from build123d import *

# Parameters (mm, degrees)
F0_R     = 65
F1_DEPTH = 174
F2_SIZE2 = 60
F2_SIZE  = 7
F3_R     = 1
F4_R     = 10
F5_R     = 66.5
F5_R_2   = 65
F6_DEPTH = 6
F7_R     = 1


with BuildPart() as f1:
    # F0 (on Top) → F1 (new body)
    with BuildSketch(Plane.XY):
        Circle(F0_R)
    extrude(amount=-F1_DEPTH)

    # F2
    f2_edges = [f1.edges().sort_by_distance(p)[0] for p in [
        (-65, 0, -174),
    ]]
    f2_side = f1.faces().sort_by_distance((-65, 0, -87))[0]
    chamfer(f2_edges, length=F2_SIZE, length2=F2_SIZE2, reference=f2_side)

    # F3
    f3_edges = [f1.edges().sort_by_distance(p)[0] for p in [
        (-5, 0, -174),
    ]]
    fillet(f3_edges, radius=F3_R)

    # F4
    f4_edges = [f1.edges().sort_by_distance(p)[0] for p in [
        (-65, 0, -167),
    ]]
    fillet(f4_edges, radius=F4_R)

    # F5 (on face) → F6 (join)
    with BuildSketch(Plane.XY):
        Circle(F5_R)
        Circle(F5_R_2, mode=Mode.SUBTRACT)
        Circle(F5_R_2)
    extrude(amount=F6_DEPTH)

    # F7
    f7_edges = [f1.edges().sort_by_distance(p)[0] for p in [
        (-66.5, 0, 6),
        (-66.5, 0, 0),
    ]]
    fillet(f7_edges, radius=F7_R)


solid = f1.part
Check sheet for the modelled part. Datum: model origin and axes. Units: mm. A direction names the side the tool comes from. Coordinates: 2 decimals unless noted, no trailing zeros. Write each loop counter-clockwise with the first axis right and the second up, starting at its lowest first coordinate (ties: lowest second). Pieces come first, ordered by that corner, then holes.
Item 1: Scan lines: probe 1 along X at (y, z) = (-0.5, -90); probe 2 along Z at (x, y) = (56.5, 32.5); probe 3 along Y at (x, z) = (7, -33). Record each from-to range of solid material in increasing order.
Numbers:
probe 1: x = -65 to 65
probe 2: z = 0 to 6
probe 3: y = -64.62 to 64.62
Item 2: Depth check by flat-ended pin: pin 1 Ø1.5 at (x, z) = (24, -62) entering from +Y; pin 2 Ø10 at (y, z) = (43.5, -106.5) entering from -X; pin 3 Ø4 at (x, z) = (45.5, -88.5) entering from -Y. Enter the tip coordinate at first touch or a pass-through.
Numbers:
pin 1: stops at y = 60.7
pin 2: stops at x = -52.37
pin 3: stops at y = -48.3
Item 3: Cross-section at A-A on z = -122. Record the boundary of the cut face in (x, y).
Numbers:
outline: circle Ø130 at (0, 0)
Item 4: Access from +Z, -Z, +X, -X, +Y, -Y to the whole of each face (thin tool, end or side, straight path). Record for faces 1 (the face through (-14.091, -63.454, -77.943)), 2 (the face through (0, 0, -174)).
Numbers:
face 1: -Z
face 2: -Z, +X, -X, +Y, -Y
